The model under review builds one solid part; all positions refer to its coordinate system, in mm. Give positions to 0.01 mm unless a question says otherwise; leave off trailing zeros. Order: outer loops, then holes, each group sorted by start corner. A loop starts at its lowest first (then second) coordinate and runs counter-clockwise, first axis right, second up. Notation, with made-up numbers: (81, -13.5) -> (115, -13.5) arc R27 ccw to (115, 24.5) -> close; hole circle Ø8 at (-30, -33). An arc over 180 degrees is marked (long way). Answer as a JSON object with one key per item and string values. Group by question number.
from build123d import *

# Parameters (mm, degrees)
EXTRUDE_1_DEPTH = 130


with BuildPart() as part:
    # 草图1 → 凸台-拉伸1 (new body)
    with BuildSketch(Plane(origin=(0, 0.070410314, -10.430830946), x_dir=(1, 0, 0), z_dir=(0, -0.006750057654754126, 0.9999772181013213))):
        Polygon((-8.5, 9.735119508), (-0.5, 9.735119508), (-0.5, 24.735119508), (-20.5, 24.735119508), (-20.5, 14.735119508), (-8.5, 14.735119508), align=None)
        Polygon((-0.5, 24.735119508), (-0.5, 9.735119508), (7.5, 9.735119508), (7.5, 14.735119508), (19.5, 14.735119508), (19.5, 24.735119508), (10.2499492, 24.735119508), (10.2499492, 22.735119508), (10.2499492, 17.735119508), (4.2499492, 17.735119508), (4.2499492, 22.735119508), (4.2499492, 24.735119508), align=None)
    extrude(amount=-EXTRUDE_1_DEPTH)


solid = part.part
1. For pin 1 (4 mm diameter, centred on x = 8.5, z = -108, fed in from -Y); pin 2 (1 mm diameter, centred on y = 12, z = -96.5, fed in from +X); pin 3 (1.8 mm diameter, centred on y = 12.5, z = -45, fed in from -X); pin 4 (1 mm diameter, centred on x = 8.5, y = 13.5, fed in from +Z), all flat-tipped, find the tip position at first contact; note any pin that passes through.
2. Take a section at A-A on y = 22.25. Give the boundary of the cut face in (x, z).
3. Draft analysis for pull direction X (two halves, no side actions). For faces 1 (the flat face through (10.25, 22, -74)), 2 (the flat face through (7.5, 13, -74)), 3 (the flat face through (-8.5, 13, -74)), state which applies: pulls with the +X half, pulls with the -X half, needs draft (parallel to the pull), parting line crosses it, or undercut.
4. Take a section at C-C on z = -116.5. Give the boundary of the cut face in (x, y), plus the area to 3 significant figures.
5. For probe 1 along X at (y, z) = (24, -19); probe 2 along X at (y, z) = (14.75, -115); probe 3 along Z at (x, y) = (2.5, 19.5), list the stretches that pass through material, from the lowest coordinate up. Write a range as [from, to].
6. Take a section at B-B on x = 16.5. Give the boundary of the cut face in (y, z).
7. Take a section at D-D on y = 13. Give the boundary of the cut face in (x, z).
Checks:
{
 "1": {"pin 1": "stops at y = 10.45", "pin 2": "stops at x = 7.5", "pin 3": "stops at x = -8.5", "pin 4": "passes through"},
 "2": {"outline": "(-20.5, -140.28) -> (4.25, -140.28) -> (4.25, -10.28) -> (-20.5, -10.28) -> close; (10.25, -140.28) -> (19.5, -140.28) -> (19.5, -10.28) -> (10.25, -10.28) -> close"},
 "3": {"face 1": "undercut", "face 2": "pulls with the +X half", "face 3": "pulls with the -X half"},
 "4": {"outline": "(-20.5, 15.52) -> (-8.5, 15.52) -> (-8.5, 10.52) -> (7.5, 10.52) -> (7.5, 15.52) -> (19.5, 15.52) -> (19.5, 25.52) -> (10.25, 25.52) -> (10.25, 18.52) -> (4.25, 18.52) -> (4.25, 25.52) -> (-20.5, 25.52) -> close", "area": "438 mm2"},
 "5": {"probe 1": "x = [-20.5, 4.25], [10.25, 19.5]", "probe 2": "x = [-8.5, 7.5]", "probe 3": "z = [-140.3, -10.3]"},
 "6": {"outline": "(14.81, -10.33) -> (15.68, -140.33) -> (25.68, -140.26) -> (24.8, -10.26) -> close"},
 "7": {"outline": "(-8.5, -140.35) -> (7.5, -140.35) -> (7.5, -10.34) -> (-8.5, -10.34) -> close"}
}
